Design review of the part shown in the three views and the two pictorial views. Dimensions are in mm from the part's minimum x, y and z. Round coordinates to 2 decimals unless told otherwise and drop trailing zeros. Write each loop counter-clockwise with the first axis right and the second up, starting at its lowest first coordinate (ties: lowest second). Pieces come first, ordered by that corner, then holes. Notation, with made-up numbers: (-15.75, -12.75) - (39.25, -12.75) arc R17 cw to (39.25, 19.25) - close; hole circle Ø9 at (22.25, 30.25). An arc over 180 degrees is marked (long way). One line per item, written item: value. Start each with the question number.
Q1. Add section C-C on y = 37. Write out the cut boundary in (x, z), and give its area (3 significant figures).
Q2. Add section D-D on x = 292. Write out the cut boundary in (y, z), and give its area (3 significant figures).
Q3. Add section A-A on z = 40.5. Write out the cut boundary in (x, y), and give its area (3 significant figures).
Q4. Add section B-B on x = 72.5. Write out the cut boundary in (y, z), and give its area (3 significant figures).
Q5. For probe 1 along Z at (x, y) = (297.5, 21); probe 2 along Y at (x, z) = (36.5, 19.5), list the stretches that pass through material, from the lowest coordinate up.
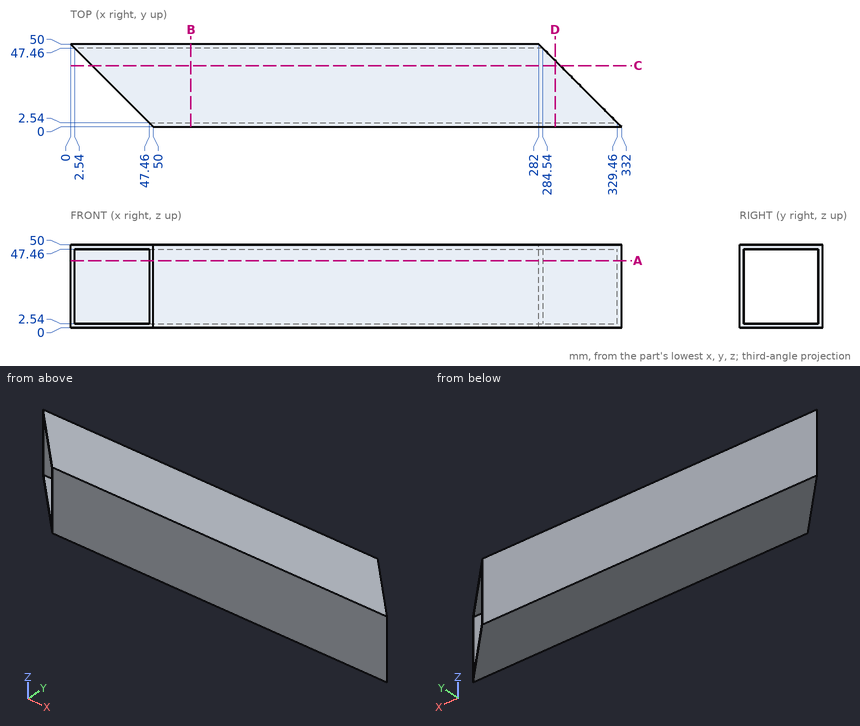
Result set:
1. outline: (13, 0) - (295, 0) - (295, 2.54) - (13, 2.54) - close; (13, 47.46) - (295, 47.46) - (295, 50) - (13, 50) - close
1. area: 1,430 mm^2
2. outline: (0, 0) - (40, 0) - (40, 2.54) - (2.54, 2.54) - (2.54, 47.46) - (40, 47.46) - (40, 50) - (0, 50) - close
2. area: 317 mm^2
3. outline: (0, 50) - (2.54, 47.46) - (284.54, 47.46) - (282, 50) - close; (47.46, 2.54) - (50, 0) - (332, 0) - (329.46, 2.54) - close
3. area: 1,430 mm^2
4. outline: (0, 0) - (50, 0) - (50, 50) - (0, 50) - close; hole (2.54, 2.54) - (47.46, 2.54) - (47.46, 47.46) - (2.54, 47.46) - close
4. area: 482 mm^2
5. probe 1: z = 0 to 2.54, 47.46 to 50
5. probe 2: y = 47.46 to 50
